Study the drawing (mm; zero at the part's minimum x, y, z) and answer. A direction names the side the tool comes from. Coordinates: 2 decimals unless noted, no trailing zeros. Loops run counter-clockwise (first coordinate to the right, second up) from the corner with the lowest first, then second, coordinate; pieces in that order, holes last. Notation, with made-up numbers: (19.5, 7.5) - (39.5, 7.5) arc R31 cw to (39.5, 45.5) - close; hole circle Ø3 at (58.25, 66.25). An arc over 180 degrees is marked (long way). Use CSV: the item, a comma, the result in double quotes.
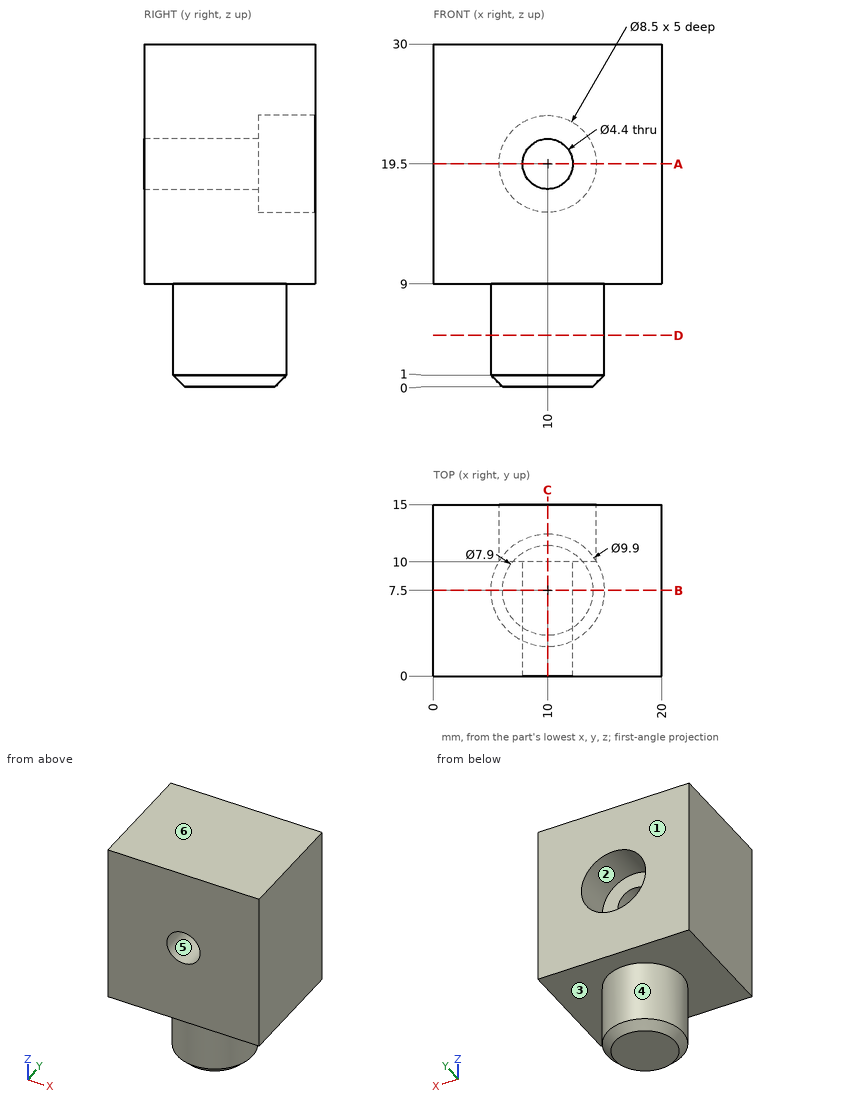
Q1. For a pull along Z with two mould halves and no side action, classify the marked faces 4, 5 and 6 as +Z half, -Z half, draft (parallel to the pull), parting line (faces both ways), or undercut.
Reported:
face 4,"draft"
face 5,"undercut"
face 6,"+Z half"
Q2. The part is cut by section D-D on z = 4.5. Determine the outline of the cut face in (x, y), and give its area (3 significant figures).
Reported:
outline,"circle Ø9.9 at (10, 7.5)"
area,"77.0 mm²"
Q3. The part is cut by section A-A on z = 19.5. Determine the outline of the cut face in (x, y).
Reported:
outline,"(0, 0) - (7.8, 0) - (7.8, 10) - (5.75, 10) - (5.75, 15) - (0, 15) - close; (12.2, 0) - (20, 0) - (20, 15) - (14.25, 15) - (14.25, 10) - (12.2, 10) - close"
Q4. The part is cut by section B-B on y = 7.5. Determine the outline of the cut face in (x, z).
Reported:
outline,"(0, 9) - (5.05, 9) - (5.05, 1) - (6.05, 0) - (13.95, 0) - (14.95, 1) - (14.95, 9) - (20, 9) - (20, 30) - (0, 30) - close; hole circle Ø4.4 at (10, 19.5)"
Q5. Given P1, Ø5, axis at x = 10, z = 19.5, coming from the +Y side; P2, Ø3, axis at x = 15, y = 10, coming from the -Z side; P3, Ø4, axis at x = 5.5, y = 12.5, coming from the -Z side, each flat-ended and moving along its own axis, determine where each tip first touches the part or whether it passes through.
Reported:
P1,"stops at y = 10"
P2,"stops at z = 0.14"
P3,"stops at z = 0.78"
Q6. Find the intervals of material crossed by probe 1 along X at (y, z) = (12.25, 19.5); probe 2 along X at (y, z) = (2.5, 19.5); probe 3 along Y at (x, z) = (13, 22.25), in increasing order. Write a range as [from, to].
Reported:
probe 1,"x = [0, 5.75], [14.25, 20]"
probe 2,"x = [0, 7.8], [12.2, 20]"
probe 3,"y = [0, 10]"
Q7. A tool of negligible diameter and unlimited length cuts with its end or side. For the marked faces 1, 2 and 3, from which of +Z, -Z, +X, -X, +Y, -Y can it reach the whole face along a straight path? Write none if from no direction.
Reported:
face 1,"+Z, -Z, +X, -X, +Y"
face 2,"+Y"
face 3,"-Z"
Q8. The part is cut by section C-C on x = 10. Determine the outline of the cut face in (y, z).
Reported:
outline,"(0, 9) - (2.55, 9) - (2.55, 1) - (3.55, 0) - (11.45, 0) - (12.45, 1) - (12.45, 9) - (15, 9) - (15, 15.25) - (10, 15.25) - (10, 17.3) - (0, 17.3) - close; (0, 21.7) - (10, 21.7) - (10, 23.75) - (15, 23.75) - (15, 30) - (0, 30) - close"
